from build123d import *

# Parameters (mm, degrees)
F0_R     = 73.968318151
F2_DEPTH = 25.4
F1_R     = 52.9945680325
F3_DEPTH = 39.624
F5_R     = 5.5188922036
F6_R     = 12.8827349719
F6_R_2   = 12.7839169131
F6_R_3   = 10.9478367458
F6_R_4   = 6.1315337815
F6_R_5   = 5.5897287033
F6_R_6   = 6.4139336727
F6_R_7   = 8.3020391009
F7_DEPTH = 70.866
F8_R     = 10.5053608139
F9_DEPTH = 50.546


with BuildPart() as f2:
    # F0 (on Top) → F2 (new body)
    with BuildSketch(Plane.XY):
        Circle(F0_R)
    extrude(amount=F2_DEPTH)

    # F1 (on face) → F3 (join)
    with BuildSketch(Plane.XY):
        Circle(F1_R)
    extrude(amount=F3_DEPTH)

    # F5
    f5_edges = [f2.edges().sort_by_distance(p)[0] for p in [
        (-52.994568, 0, 25.4),
        (52.994568, 0, 32.512),
        (-52.994568, 0, 39.624),
        (73.968318, 0, 12.7),
        (-73.968318, 0, 0),
        (-73.968318, 0, 25.4),
    ]]
    fillet(f5_edges, radius=F5_R)

    # F6 (on face) → F7 (cut)
    with BuildSketch(Plane.XY.offset(39.624)):
        with Locations((0, 22.9584183544)):
            Circle(F6_R)
        with Locations((0, -22.6955935359)):
            Circle(F6_R_2)
        with Locations((-20.5665808171, 0)):
            Circle(F6_R_3)
        with Locations((-27.7332775295, -22.6955935359)):
            Circle(F6_R_4)
        with Locations((-30.5117629468, 22.9584183544)):
            Circle(F6_R_5)
        with Locations((23.4740655869, 22.9584183544)):
            Circle(F6_R_6)
        with Locations((25.338197127, -22.6955935359)):
            Circle(F6_R_7)
    extrude(amount=-F7_DEPTH, mode=Mode.SUBTRACT)

    # F8 (on face) → F9 (cut)
    with BuildSketch(Plane.XY.offset(39.624)):
        with Locations((19.8444724083, 0)):
            Circle(F8_R)
    extrude(amount=-F9_DEPTH, mode=Mode.SUBTRACT)


solid = f2.part
Could you check a few things on this model? Use its own coordinates, in mm. Round coordinates to 2 decimals unless told otherwise and drop trailing zeros. Order: outer loops, then holes, each group sorted by start corner. A loop starts at its lowest first (then second) coordinate and runs counter-clockwise, first axis right, second up.
(1) Imagine slicing it at B-B (x = 0). Write out the boundary of the cut face in (y, z).
Response values:
outline: (-73.97, 5.52) arc R5.52 ccw to (-68.45, 0) - (-35.48, 0) - (-35.48, 39.62) - (-47.48, 39.62) arc R5.52 ccw to (-52.99, 34.11) - (-52.99, 30.92) arc R5.52 cw to (-58.51, 25.4) - (-68.45, 25.4) arc R5.52 ccw to (-73.97, 19.88) - close; (-9.91, 0) - (10.08, 0) - (10.08, 39.62) - (-9.91, 39.62) - close; (35.84, 0) - (68.45, 0) arc R5.52 ccw to (73.97, 5.52) - (73.97, 19.88) arc R5.52 ccw to (68.45, 25.4) - (58.51, 25.4) arc R5.52 cw to (52.99, 30.92) - (52.99, 34.11) arc R5.52 ccw to (47.48, 39.62) - (35.84, 39.62) - close
(2) Imagine slicing it at A-A (y = 0). Write out the boundary of the cut face in (x, z).
Response values:
outline: (-73.97, 5.52) arc R5.52 ccw to (-68.45, 0) - (-31.51, 0) - (-31.51, 39.62) - (-47.48, 39.62) arc R5.52 ccw to (-52.99, 34.11) - (-52.99, 30.92) arc R5.52 cw to (-58.51, 25.4) - (-68.45, 25.4) arc R5.52 ccw to (-73.97, 19.88) - close; (-9.62, 0) - (9.34, 0) - (9.34, 39.62) - (-9.62, 39.62) - close; (30.35, 0) - (68.45, 0) arc R5.52 ccw to (73.97, 5.52) - (73.97, 19.88) arc R5.52 ccw to (68.45, 25.4) - (58.51, 25.4) arc R5.52 cw to (52.99, 30.92) - (52.99, 34.11) arc R5.52 ccw to (47.48, 39.62) - (30.35, 39.62) - close
(3) Imagine slicing it at C-C (z = 22.5). Count the separate pieces of the cut face and the enclosed holes in it, plus the area to 3 significant figures.
Response values:
separate pieces: 1
enclosed holes: 8
area: 14,600 mm2
(4) If we mould it in two halves opening along Y, with no side actions, what happens to faces 1 (the cylindrical face through (-11.488, -51.734, 32.49)), 2 (the cylindrical face through (-10.454, -4.193, 20.089)), 3 (the flat face through (50, 31, 25.4))? For each: released by +Y, released by -Y, zero draft, split by the parting line, or undercut.
Response values:
face 1: split by the parting line
face 2: undercut
face 3: zero draft
(5) I'm going to push flat-ended pins straight in: pin 1 (8 mm diameter, centred on x = -55, y = -56, fed in from -Z); pin 2 (10 mm diameter, centred on y = 16.5, z = 25.5, fed in from -X); pin 3 (12 mm diameter, centred on y = -46.5, z = 12, fed in from +X); pin 4 (4 mm diameter, centred on x = -46.5, y = 23.5, fed in from +Z). Where does each tip first touch, or does it pass through?
Response values:
pin 1: passes through
pin 2: stops at x = -72.48
pin 3: stops at x = 61.9
pin 4: stops at z = 38.96
(6) Please list where these lines run through material, in increasing order: line 1 along X through (y, z) = (-0.5, 34); line 2 along Y through (x, z) = (23.5, 13.5); line 3 along Y through (x, z) = (0, 22).
Response values:
line 1: x = -52.99 to -31.5, -9.63 to 9.35, 30.34 to 52.99
line 2: y = -70.14 to -30.79, -14.6 to -9.85, 9.85 to 16.54, 29.37 to 70.14
line 3: y = -73.55 to -35.48, -9.91 to 10.08, 35.84 to 73.55
